Answer from the drawing. Dimensions are ordinates in mm from the lowest x, y and z of the part. A direction names the side the tool comes from. Give positions to 0.01 mm unless a question says otherwise; leave off trailing zeros. Loops run counter-clockwise (first coordinate to the right, second up) from the corner with the lowest first, then second, coordinate; pieces in that order, holes last. Notation, with made-up numbers: (45, 47) -> (67, 47) arc R16 cw to (67, 55) -> close; hole circle Ø6 at (77, -21.75). An arc over 180 degrees is marked (long way). Answer as CSV lines item,"result". Start each with the question number.
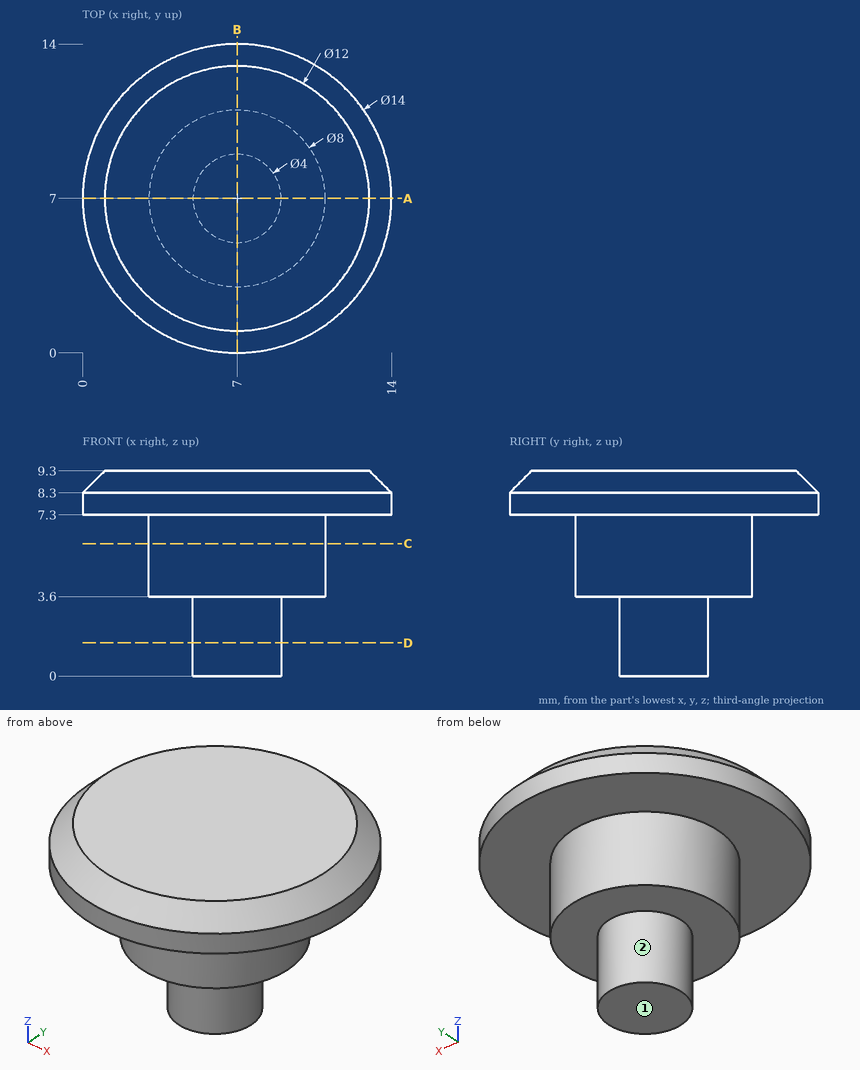
(1) Find section D-D on z = 1.5. Write down the section's boundary in (x, y), then the cut area to 3 significant figures.
(2) This flat-tipped pin is pushed along its axis until it touches: P1, Ø3, axis at y = 12, z = 4, coming from the -X side. Where does it stop, or does it pass through?
(3) Find section A-A on y = 7. Write down the section's boundary in (x, z).
(4) Find the intervals of material crossed by line 1 along Z through (x, y) = (10.75, 5); line 2 along Z through (x, y) = (4.5, 6.25); line 3 along X through (y, z) = (6.25, 4.25), in increasing order. Write a range as from..to.
(5) Find section C-C on z = 6. Write down the section's boundary in (x, y).
(6) A tool of negligible diameter and unlimited length cuts with its end or side. For the marked faces 1 and 2, from which of +Z, -Z, +X, -X, +Y, -Y can it reach the whole face along a straight path? Write none if from no direction.
Answer block:
1,outline,"circle Ø4 at (7, 7)"
1,area,"12.6 mm2"
2,P1,"stops at x = 5.06"
3,outline,"(0, 7.3) -> (3, 7.3) -> (3, 3.6) -> (5, 3.6) -> (5, 0) -> (9, 0) -> (9, 3.6) -> (11, 3.6) -> (11, 7.3) -> (14, 7.3) -> (14, 8.3) -> (13, 9.3) -> (1, 9.3) -> (0, 8.3) -> close"
4,line 1,"z = 7.3..9.3"
4,line 2,"z = 3.6..9.3"
4,line 3,"x = 3.07..10.93"
5,outline,"circle Ø8 at (7, 7)"
6,face 1,"-Z, +X, -X, +Y, -Y"
6,face 2,"-Z"
